Can you work these out from the model? Positions are in its coordinate system, mm. Face numbers are marked on the shaded views. A direction names the side the tool comes from. Coordinates: 2 decimals unless noted, no trailing zeros. Order: outer loops, then holes, each group sorted by start corner. A loop starts at its lowest first (then second) coordinate and runs counter-clockwise, first axis right, second up. Notation, with made-up numbers: (7.5, 49) -> (33.5, 49) arc R24 cw to (33.5, 62) -> close; hole circle Ø2 at (65.5, -33). An arc over 180 degrees is marked (long way). Return JSON: item names as keys, results as strings. Group by question number.
1) If we section it at A-A, the plane z = 5.25: State how many separate pieces and enclosed holes the cut face has, then the cut area to 3 significant figures.
2) If I drill on probe 1 along X at (y, z) = (-4, 4.25); probe 2 along Y at (x, z) = (0, 6.7); probe 3 along X at (y, z) = (0.5, 3.5), over which ranges is the centre line in solid material (lowest first)? Write a range as from..to.
3) For the marked faces 1 and 2, which set-ups out of +Z, -Z, +X, -X, +Y, -Y let a thin tool reach every point of the face, with its end or its side?
4) If we section it at B-B, the plane z = 1.25: Please give me the cut outline in (x, y), then the cut area to 3 significant figures.
5) Thinking about a two-plate mould opening in Y: for the marked faces 3, 4 and 5, which applies, +Y half, -Y half, draft (parallel to the pull), parting line (faces both ways), or undercut?
6) For pin 1 (3 mm diameter, centred on y = 16, z = 3, fed in from +X); pin 2 (5 mm diameter, centred on x = -21.5, y = 2, fed in from +Z); pin 3 (4 mm diameter, centred on x = -6.5, z = 0, fed in from -Y); pin 4 (3 mm diameter, centred on x = -16.5, y = 13, fed in from -Z), each with a flat end and sliding along its axis, tell me the tip position at first contact or that it passes through.
from build123d import *

# Parameters (mm, degrees)
EXTRUDE_1_DEPTH     = 5
CUT_EXTRUDE_1_DEPTH = 2.5
SKETCH_4_R          = 3.5
SKETCH_4_R_2        = 2.5
EXTRUDE_2_DEPTH     = 2.5
FILLET_1_R          = 2
FILLET_2_R          = 2
FILLET_3_R          = 2
SCALE_1_SCALE       = 2


with BuildPart() as part:
    # 草图2 → 凸台-拉伸1 (new body)
    with BuildSketch(Plane.XY):
        with BuildLine():
            Line((12.990381057, -2.5), (4.330127019, 12.5))
            ThreePointArc((4.330127019, 12.5), (0, 15), (-4.330127019, 12.5))
            Line((-4.330127019, 12.5), (-12.990381057, -2.5))
            ThreePointArc((-12.990381057, -2.5), (-12.990381057, -7.5), (-8.660254038, -10))
            Line((-8.660254038, -10), (8.660254038, -10))
            ThreePointArc((8.660254038, -10), (12.990381057, -7.5), (12.990381057, -2.5))
        make_face()
    extrude(amount=EXTRUDE_1_DEPTH)

    # 草图3 → 切除-拉伸1 (cut)
    with BuildSketch(Plane.XY.offset(5)):
        with BuildLine():
            Line((11.258330249, -3.5), (2.598076211, 11.5))
            ThreePointArc((2.598076211, 11.5), (0, 13), (-2.598076211, 11.5))
            Line((-2.598076211, 11.5), (-11.258330249, -3.5))
            ThreePointArc((-11.258330249, -3.5), (-11.258330249, -6.5), (-8.660254038, -8))
            Line((-8.660254038, -8), (8.660254038, -8))
            ThreePointArc((8.660254038, -8), (11.258330249, -6.5), (11.258330249, -3.5))
        make_face()
    extrude(amount=-CUT_EXTRUDE_1_DEPTH, mode=Mode.SUBTRACT)

    # 草图4 → 凸台-拉伸2 (add)
    with BuildSketch(Plane.XY.offset(2.5)):
        Circle(SKETCH_4_R)
        Circle(SKETCH_4_R_2, mode=Mode.SUBTRACT)
    extrude(amount=EXTRUDE_2_DEPTH)

    # 圆角1
    fillet_1_edges = [part.edges().sort_by_distance(p)[0] for p in [
        (0, 15, 5),
        (-8.660254038, 5, 5),
        (-12.990381057, -7.5, 5),
        (0, -10, 5),
        (12.990381057, -7.5, 5),
        (8.660254038, 5, 5),
    ]]
    fillet(fillet_1_edges, radius=FILLET_1_R - 0.0001)  # a hair under: the kernel refuses the full size

    # 圆角2
    fillet_2_edges = [part.edges().sort_by_distance(p)[0] for p in [
        (11.258330249, -6.5, 2.5),
        (0, -8, 2.5),
        (-11.258330249, -6.5, 2.5),
        (-6.92820323, 4, 2.5),
        (0, 13, 2.5),
        (6.92820323, 4, 2.5),
        (-3.5, 0, 2.5),
    ]]
    fillet(fillet_2_edges, radius=FILLET_2_R)

    # 圆角3
    fillet_3_edges = [part.edges().sort_by_distance(p)[0] for p in [
        (0, -10, 0),
        (-12.990381057, -7.5, 0),
        (-8.660254038, 5, 0),
        (0, 15, 0),
        (8.660254038, 5, 0),
        (12.990381057, -7.5, 0),
    ]]
    fillet(fillet_3_edges, radius=FILLET_3_R)


with BuildPart() as part_1:
    # 缩放比例1: scaled about (0, 0, 1.925767513)
    add(part.part.scale(SCALE_1_SCALE).moved(Location((0, 0, -1.925767513))))


solid = part_1.part
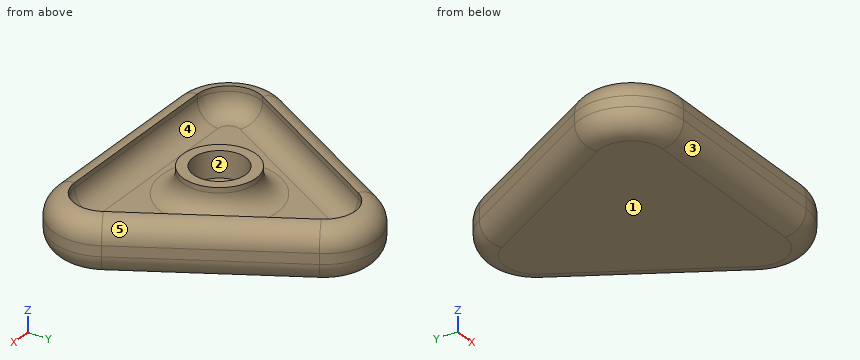
Result sheet:
{
 "1": {"separate pieces": "2", "enclosed holes": "2", "area": "744 mm2"},
 "2": {"probe 1": "x = -25.4..-19.44, -7.12..-3, 3..7.12, 19.44..25.4", "probe 2": "y = -19.02..-15.98, -7.02..-5, 5..7.02, 25.98..29.02", "probe 3": "x = -22.81..-15.64, -9.19..-4.97, 4.97..9.19, 15.64..22.81"},
 "3": {"face 1": "-Z, +X, -X, +Y, -Y", "face 2": "+Z"},
 "4": {"outline": "(-25.91, -5.04) arc R9.91 ccw to (-17.32, -19.91) -> (17.32, -19.91) arc R9.91 ccw to (25.91, -5.04) -> (8.59, 24.96) arc R9.91 ccw to (-8.59, 24.96) -> close", "area": "1,860 mm2"},
 "5": {"face 3": "-Y half", "face 4": "undercut", "face 5": "+Y half"},
 "6": {"pin 1": "stops at x = 14.72", "pin 2": "stops at z = 7.91", "pin 3": "stops at y = -20", "pin 4": "stops at z = -0.2"}
}
